Verification items for the finished model (mm, model axes). Face numbers are marked on the shaded views. A direction names the side the tool comes from. Give positions to 0.01 mm unless a question says otherwise; leave off trailing zeros. Write each loop counter-clockwise with the first axis right and the second up, starting at its lowest first coordinate (ties: lowest second). Pieces come first, ordered by that corner, then holes. Notation, with made-up numbers: M 35,-10.75 L 64,-10.75 A33 cw 64,26.25 Z; hole C -38,77.25 d5. An arc over 180 degrees is marked long. Answer as a JSON object with one key per item and string values.
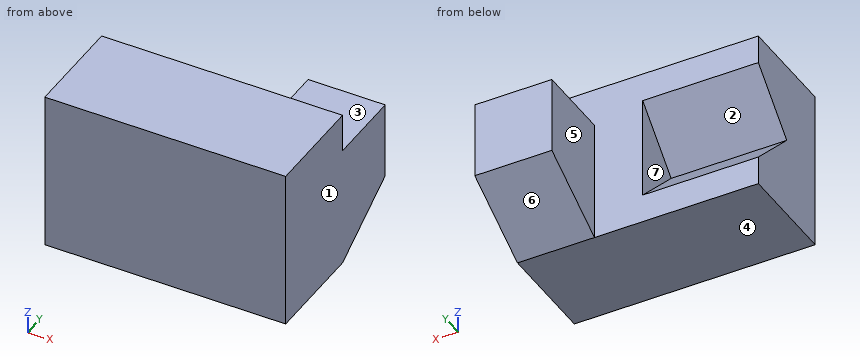
```python
from build123d import *

# Parameters (mm, degrees)
SKETCH2_W           = 75
SKETCH2_H           = 50
BOSS_EXTRUDE1_DEPTH = 32
CUT_EXTRUDE1_DEPTH  = 36
SKETCH5_W           = 24
SKETCH5_H           = 24
BOSS_EXTRUDE3_DEPTH = 24
BOSS_EXTRUDE4_DEPTH = 24


with BuildPart() as part:
    # Sketch2 → Boss-Extrude1 (new body)
    with BuildSketch(Plane(origin=(0, 0, 0), x_dir=(1, 0, 0), z_dir=(0, 1, 0))):
        with Locations((1.812039309, 0.877582126)):
            Rectangle(SKETCH2_W, SKETCH2_H)
    extrude(amount=BOSS_EXTRUDE1_DEPTH)

    # Sketch4 → Cut-Extrude1 (cut)
    with BuildSketch(Plane.ZY.offset(35.687960691)):
        Polygon((-16.877582126, 32), (-0.877582126, 16), (15.122417874, 32), align=None)
    extrude(amount=-CUT_EXTRUDE1_DEPTH, mode=Mode.SUBTRACT)

    # Sketch5 → Boss-Extrude3 (add)
    with BuildSketch(Plane(origin=(0, 32, 0), x_dir=(1, 0, 0), z_dir=(0, 1, 0))):
        with Locations((27.312039309, -0.122417874)):
            Rectangle(SKETCH5_W, SKETCH5_H)
    extrude(amount=BOSS_EXTRUDE3_DEPTH)

    # Sketch6 → Boss-Extrude4 (add)
    with BuildSketch(Plane(origin=(39.312039309, 0, 0), x_dir=(0, 0, -1), z_dir=(1, 0, 0))):
        Polygon((11.877582126, 56), (25.877582126, 32), (11.877582126, 32), align=None)
    extrude(amount=-BOSS_EXTRUDE4_DEPTH)


solid = part.part
```
1) Go/stop test with flat-tipped pins: pin 1 (2 mm diameter, centred on x = 7, z = 7, fed in from +Y); pin 2 (13 mm diameter, centred on y = 26, z = 6.5, fed in from -X); pin 3 (19 mm diameter, centred on x = 30, y = 47.5, fed in from +Z); pin 4 (19 mm diameter, centred on y = 39.5, z = -9, fed in from -X). Record where each tip stops, or that it passes through.
Completed:
{"pin 1": "stops at y = 32", "pin 2": "stops at x = -35.69", "pin 3": "stops at z = 12.12", "pin 4": "stops at x = 0.31"}
2) Section check D-D on x = -1.5. Record the boundary of the cut face in (y, z).
Completed:
{"outline": "M 0,-25.88 L 32,-25.88 L 32,-16.88 L 16,-0.88 L 32,15.12 L 32,24.12 L 0,24.12 Z"}
3) Section check C-C on y = 31. Record the boundary of the cut face in (x, z).
Completed:
{"outline": "M -35.69,-25.88 L 39.31,-25.88 L 39.31,24.12 L -35.69,24.12 L -35.69,14.12 L 0.31,14.12 L 0.31,-15.88 L -35.69,-15.88 Z"}
4) Release check for a two-part mould opening along Z. For the marked faces 1, 2, 3 and 4 record: pulls with the +Z half, pulls with the -Z half, needs draft (parallel to the pull), parting line crosses it, or undercut.
Completed:
{"face 1": "needs draft", "face 2": "undercut", "face 3": "pulls with the +Z half", "face 4": "pulls with the -Z half"}
5) Section check B-B on z = 10.5. Record the boundary of the cut face in (x, y).
Completed:
{"outline": "M -35.69,0 L 39.31,0 L 39.31,56 L 15.31,56 L 15.31,32 L 0.31,32 L 0.31,27.38 L -35.69,27.38 Z"}
6) Thickness scan on L1, parallel to Z at x = -19.5, y = 26.5; L2, parallel to X at y = 37, z = 6.5; L3, parallel to Y at x = -7.5, z = -22. Record the ranges inside material, lowest first.
Completed:
{"L1": "z = -25.88 to -11.38, 9.62 to 24.12", "L2": "x = 15.31 to 39.31", "L3": "y = 0 to 32"}
7) Section check A-A on x = 26. Record the boundary of the cut face in (y, z).
Completed:
{"outline": "M 0,-25.88 L 32,-25.88 L 56,-11.88 L 56,12.12 L 32,12.12 L 32,24.12 L 0,24.12 Z"}
8) Access from +Z, -Z, +X, -X, +Y, -Y to the whole of each face (thin tool, end or side, straight path). Record for the marked faces 5, 6 and 7.
Completed:
{"face 5": "+Z, -Z, -X, +Y", "face 6": "-Z, +X, -X, +Y", "face 7": "-X, +Y"}
